```python
from build123d import *

# Parameters (mm, degrees)
SKETCH3_R               = 3.69
SKETCH3_R_2             = 2.69
EXTRUDE_THIN1_DEPTH     = 3.5
SKETCH4_W               = 1
SKETCH4_H               = 1000
CUT_EXTRUDE1_DEPTH      = 4.5
CUT_EXTRUDE1_DEPTH_BACK = 4.5
FILLET1_R               = 1


with BuildPart() as part:
    # Sketch3 → Extrude-Thin1 (new body, symmetric)
    with BuildSketch(Plane(origin=(0, 0, 0), x_dir=(1, 0, 0), z_dir=(0, 1, 0))):
        Circle(SKETCH3_R)
        Circle(SKETCH3_R_2, mode=Mode.SUBTRACT)
    extrude(amount=EXTRUDE_THIN1_DEPTH, both=True)

    # Sketch4 → Cut-Extrude1 (cut, two sides)
    with BuildSketch(Plane(origin=(0, 0, 0), x_dir=(1, 0, 0), z_dir=(0, 1, 0))) as cut_extrude1_sk:
        with Locations((0, 500)):
            Rectangle(SKETCH4_W, SKETCH4_H)
    extrude(amount=CUT_EXTRUDE1_DEPTH, mode=Mode.SUBTRACT)
    extrude(cut_extrude1_sk.sketch, amount=-CUT_EXTRUDE1_DEPTH_BACK, mode=Mode.SUBTRACT)

    # Fillet1
    fillet1_edges = [part.edges().sort_by_distance(p)[0] for p in [
        (0.5, -3.5, -3.149545438),
        (-0.5, -3.5, -3.149545438),
        (0.5, 3.5, -3.149545438),
        (-0.5, 3.5, -3.149545438),
    ]]
    fillet(fillet1_edges, radius=FILLET1_R)


solid = part.part
```
Source: CAD feature listing. Evaluate the final solid. Frame: model axes, mm. A direction names the side the tool comes from. Coordinates: 2 decimals unless noted, no trailing zeros. Loops run counter-clockwise (first coordinate to the right, second up) from the corner with the lowest first, then second, coordinate; pieces in that order, holes last. Notation, with made-up numbers: M 62.5,28 L 71.5,28 A24 ccw 71.5,56 Z; hole C -2,73.25 d8. An arc over 180 degrees is marked long. Use a Markdown table: item, result. Add a question column.
Q1. First-contact query: pin 1 (1.1 mm diameter, centred on y = -1, z = -3.5, fed in from -X); pin 2 (3 mm diameter, centred on y = 0, z = -2, fed in from -X); pin 3 (1 mm diameter, centred on y = 2.5, z = -3, fed in from +X). Flat tips, straight axial feed; report the tip coordinate or a pass-through.
Q2. Material intervals for L1, parallel to X at y = -1, z = 0; L2, parallel to Z at x = 0, y = 2; L3, parallel to Z at x = -2.25, y = 2.75, sorted ascending.
Q3. Access query for faces 1 (the flat face through (0.5, 0, -3)), 2 (the cylindrical face through (-0.785, 3.199, -3.093)), 3 (the cylindrical face through (0.785, -3.199, -3.113)), 4 (the flat face through (0, -3.5, 3)). Directions: +Z, -Z, +X, -X, +Y, -Y. A direction counts if a zero-diameter tool reaches every point of the face in a straight line with its end or side. Return the directions, or none.
Q4. Section query B-B, the plane x = 1.75. Return loops of the section in (y, z), and give its area (3 significant figures).
Q5. Section query C-C, the plane y = 1.5. Return loops of the section in (x, z), and give its area (3 significant figures).
Q6. Draft query along Z for faces 5 (the flat face through (0, 3.5, 3)), 6 (the cylindrical face through (-0.111, -0.049, 2.688)), 7 (the cylindrical face through (-0.155, 0.049, 3.687)). Return one class per face: pulls with the +Z half, pulls with the -Z half, needs draft (parallel to the pull), parting line crosses it, or undercut.
Q7. Section query A-A, the plane z = 0. Return loops of the section in (x, y).
Q8. Section query D-D, the plane z = -3. Return loops of the section in (x, y), and give its area (3 significant figures).
Result:
| question | item | result |
|---|---|---|
| 1 | pin 1 | stops at x = -2.22 |
| 1 | pin 2 | stops at x = -3.66 |
| 1 | pin 3 | stops at x = 2.71 |
| 2 | L1 | x = -3.69 to -2.69, 2.69 to 3.69 |
| 2 | L2 | z = 2.69 to 3.69 |
| 2 | L3 | z = -2.92 to -1.47, 1.47 to 2.92 |
| 3 | face 1 | -Z, +Y, -Y |
| 3 | face 2 | -Z, +Y |
| 3 | face 3 | -Z, -Y |
| 3 | face 4 | +Z, -Z, +X, -X, -Y |
| 4 | outline | M -3.5,-3.25 L 3.5,-3.25 L 3.5,-2.04 L -3.5,-2.04 Z; M -3.5,2.04 L 3.5,2.04 L 3.5,3.25 L -3.5,3.25 Z |
| 4 | area | 16.9 mm2 |
| 5 | outline | M -0.5,-3.66 L -0.5,-2.64 A2.69 cw long 0.5,-2.64 L 0.5,-3.66 A3.69 ccw long Z |
| 5 | area | 19.0 mm2 |
| 6 | face 5 | needs draft |
| 6 | face 6 | undercut |
| 6 | face 7 | parting line crosses it |
| 7 | outline | M -3.69,-3.5 L -2.69,-3.5 L -2.69,3.5 L -3.69,3.5 Z; M 2.69,-3.5 L 3.69,-3.5 L 3.69,3.5 L 2.69,3.5 Z |
| 8 | outline | M -2.15,-3.5 L -1.5,-3.5 A1 ccw -0.5,-2.5 L -0.5,2.5 A1 ccw -1.5,3.5 L -2.15,3.5 Z; M 0.5,-2.5 A1 ccw 1.5,-3.5 L 2.15,-3.5 L 2.15,3.5 L 1.5,3.5 A1 ccw 0.5,2.5 Z |
| 8 | area | 22.2 mm2 |
